```python
from build123d import *

# Parameters (mm, degrees)
F0_R     = 9.525
F1_DEPTH = 25.4
F3_R     = 4.7625
F4_DEPTH = 25.401
F2_W     = 9.525
F2_H     = 9.525
F5_DEPTH = 11.0998
F7_DEPTH = 14.605


with BuildPart() as f1:
    # F0 (on Front) → F1 (new body)
    with BuildSketch(Plane.XZ):
        Circle(F0_R)
    extrude(amount=F1_DEPTH)

    # F3 (on Front) → F4 (cut, through all)
    with BuildSketch(Plane.XZ):
        Circle(F3_R)
    extrude(amount=F4_DEPTH, mode=Mode.SUBTRACT)

    # F2 (on Front) → F5 (cut)
    with BuildSketch(Plane.XZ):
        Rectangle(F2_W, F2_H)
    extrude(amount=F5_DEPTH, mode=Mode.SUBTRACT)

    # F6 (on face) → F7 (cut)
    with BuildSketch(Plane(origin=(0, 0, 0), x_dir=(-1, 0, 0), z_dir=(0, 1, 0))):
        Polygon((4.247856, -6.267943), (7.54897, -0.586891), (5.165556, 5.536102), (-1.107627, 7.490297), (-6.546745, 3.804146), (-7.05603, -2.746605), (-2.251981, -7.229106), align=None)
    extrude(amount=-F7_DEPTH, mode=Mode.SUBTRACT)


solid = f1.part
```
Model file for the job. Use its own axes, mm. A direction names the side the tool comes from. Give positions to 0.01 mm unless a question says otherwise; leave off trailing zeros. Loops run counter-clockwise (first coordinate to the right, second up) from the corner with the lowest first, then second, coordinate; pieces in that order, holes last. Notation, with made-up numbers: (-35.75, 56) - (-7.75, 56) arc R12 ccw to (-7.75, 60) - close; hole circle Ø4 at (43.5, 6). An arc over 180 degrees is marked (long way). One line per item, written item: value. Start each with the question number.
1. Probe L1, parallel to Z at x = 0, y = -22.75 (1 decimal); L2, parallel to Z at x = -8.25, y = -3.75; L3, parallel to Y at x = 2.75, z = 4.75 (3 decimals). List the from-to ranges inside material, lowest first. Write a range as from..to.
2. Pin check, flat tips, straight feed: pin 1 (2 mm diameter, centred on x = 5, y = -23, fed in from +Z); pin 2 (6 mm diameter, centred on y = -15.5, z = 6.5, fed in from -X); pin 3 (4 mm diameter, centred on y = -16, z = -5, fed in from -X). Stop position of each tip, or through.
3. Pull direction X, two halves, no side cores. Call faces 3 (the cylindrical face through (-7.559, -12.522, -5.796)), 4 (the flat face through (-4.4, -25.4, 2.3)), 5 (the flat face through (-2.07, -7.2, 6.5)): pulls with the +X half, pulls with the -X half, needs draft (parallel to the pull), parting line crosses it, or undercut.
4. Slice it at D-D (x = 5.25). List the corners of the cut face in (y, z) (3 decimals).
5. Slice it at B-B (z = 0). List the corners of the cut face in (x, y) (1 decimal).
6. Slice it at C-C (x = 0). List the corners of the cut face in (y, z) (1 decimal).
7. Which spindle directions (+Z, -Z, +X, -X, +Y, -Y) get a long thin tool onto all of the face, cutting with end or side? Do faces 1 (the cylindrical face through (-3.78, -19.93, -2.9)), 2 (the flat face through (1, -14.605, -5)). Say none if no direction does.
8. Slice it at A-A (y = -5.75). List the corners of the cut face in (x, z) (3 decimals).
Solution:
1. L1: z = -9.5..-4.8, 4.8..9.5
1. L2: z = -4.76..4.76
1. L3: y = -25.4..-14.605
2. pin 1: stops at z = 8.64
2. pin 2: stops at x = -8.86
2. pin 3: stops at x = -9.04
3. face 3: parting line crosses it
3. face 4: needs draft
3. face 5: undercut
4. outline: (-25.4, -7.948) - (0, -7.948) - (0, -4.432) - (-14.605, -4.432) - (-14.605, 4.683) - (0, 4.683) - (0, 7.948) - (-25.4, 7.948) - close
5. outline: (-9.5, -25.4) - (-4.8, -25.4) - (-4.8, -14.6) - (-7.3, -14.6) - (-7.3, 0) - (-9.5, 0) - close; (4.8, -25.4) - (9.5, -25.4) - (9.5, 0) - (6.8, 0) - (6.8, -14.6) - (4.8, -14.6) - close
6. outline: (-25.4, -9.5) - (0, -9.5) - (0, -6.9) - (-14.6, -6.9) - (-14.6, -4.8) - (-25.4, -4.8) - close; (-25.4, 4.8) - (-14.6, 4.8) - (-14.6, 7.1) - (0, 7.1) - (0, 9.5) - (-25.4, 9.5) - close
7. face 1: +Y, -Y
7. face 2: +Y
8. outline: circle Ø19.05 at (0, 0); hole (-7.549, -0.587) - (-4.248, -6.268) - (2.252, -7.229) - (7.056, -2.747) - (6.547, 3.804) - (1.108, 7.49) - (-5.166, 5.536) - close
